Part print with two shaded views. Sizes in mm from the minimum x, y, z corner. Give positions to 0.01 mm unless a question says otherwise; leave off trailing zeros. Write each loop counter-clockwise with the first axis right and the second up, starting at its lowest first coordinate (ties: lowest second). Pieces come first, ordered by that corner, then holes.
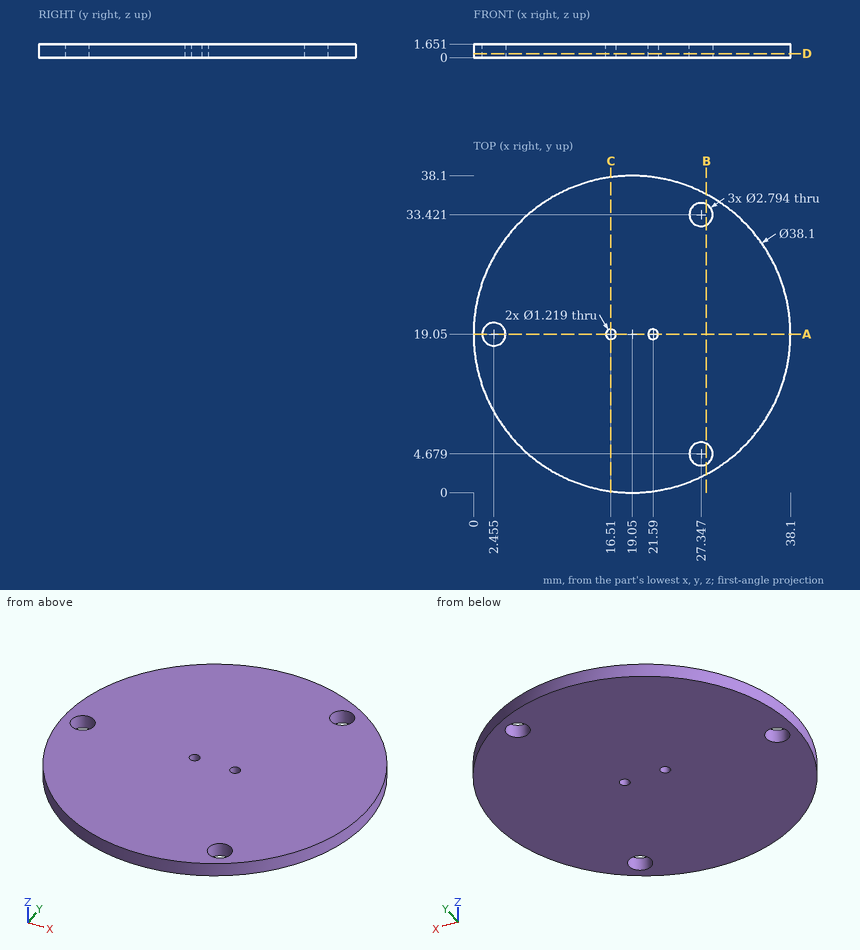
(1) Saw through at D-D, the plane z = 0.5. Give the number of separate pieces and of enclosed holes in the cut face, plus the area to 3 significant figures.
(2) Probe line 1 (X direction, y = 19, z = 0.75); line 2 (Y direction, x = 28.5, z = 1.1) (1 decimal); line 3 (Y direction, x = 21.59, z = 1.2). List the from-to ranges inside material, lowest first.
(3) Saw through at A-A, the plane y = 19.05. List the corners of the cut face in (x, z).
(4) Saw through at C-C, the plane x = 16.51. List the corners of the cut face in (y, z).
(5) Saw through at B-B, the plane x = 28. List the corners of the cut face in (y, z).
Computed values:
1. separate pieces: 1
1. enclosed holes: 5
1. area: 1,120 mm2
2. line 1: x = 0 to 1.06, 3.85 to 15.9, 17.12 to 20.98, 22.2 to 38.1
2. line 2: y = 2.5 to 3.9, 5.5 to 32.6, 34.2 to 35.6
2. line 3: y = 0.17 to 18.44, 19.66 to 37.93
3. outline: (0, 0) - (1.06, 0) - (1.06, 1.65) - (0, 1.65) - close; (3.85, 0) - (15.9, 0) - (15.9, 1.65) - (3.85, 1.65) - close; (17.12, 0) - (20.98, 0) - (20.98, 1.65) - (17.12, 1.65) - close; (22.2, 0) - (38.1, 0) - (38.1, 1.65) - (22.2, 1.65) - close
4. outline: (0.17, 0) - (18.44, 0) - (18.44, 1.65) - (0.17, 1.65) - close; (19.66, 0) - (37.93, 0) - (37.93, 1.65) - (19.66, 1.65) - close
5. outline: (2.23, 0) - (3.44, 0) - (3.44, 1.65) - (2.23, 1.65) - close; (5.91, 0) - (32.19, 0) - (32.19, 1.65) - (5.91, 1.65) - close; (34.66, 0) - (35.87, 0) - (35.87, 1.65) - (34.66, 1.65) - close
